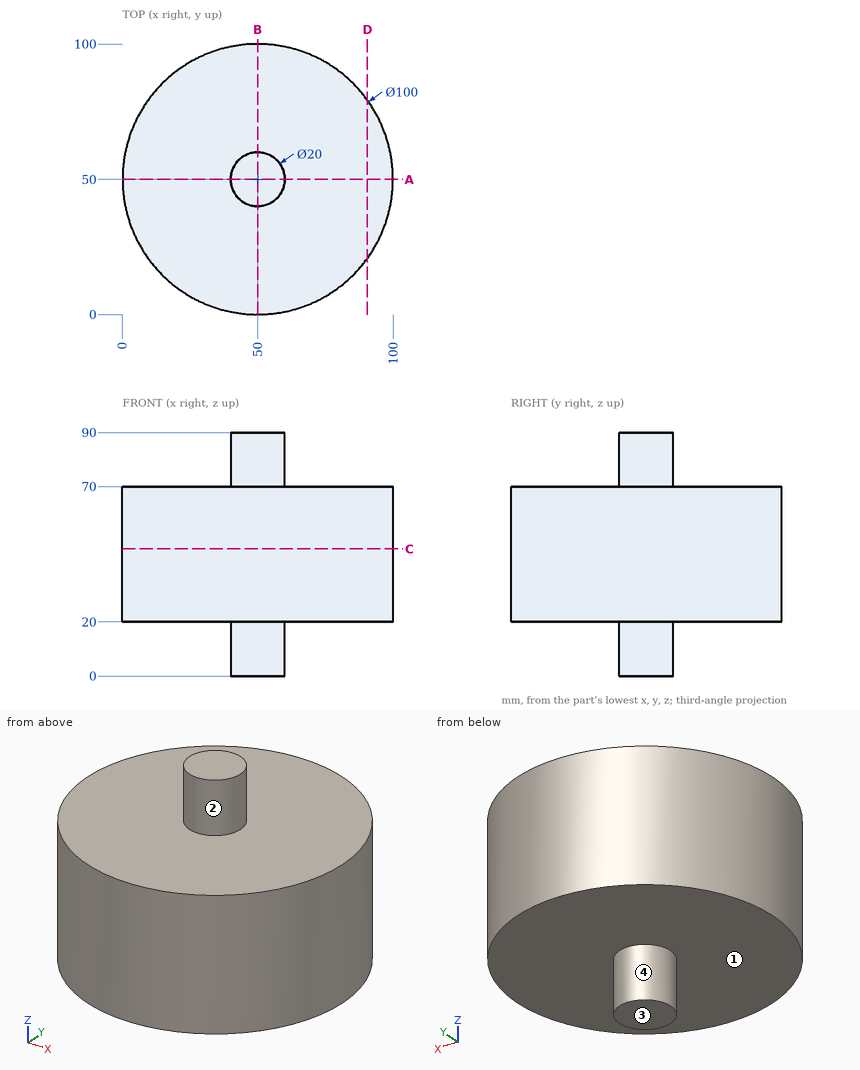
Verification items for this drawing (mm, ordinates from the low corner). A direction names the side the tool comes from. Give positions to 0.01 mm unless a question says otherwise; leave off trailing zeros. Loops run counter-clockwise (first coordinate to the right, second up) from the corner with the lowest first, then second, coordinate; pieces in that order, holes last. Notation, with made-up numbers: M 39.25,-37 L 48.25,-37 A12 ccw 48.25,-17 Z; hole C -19.75,39 d6. An arc over 180 degrees is marked long. Write item = value, one per line. Start each with the question number.
1. Draft check along X on the marked faces 1 and 2. Enter one of: +X half, -X half, draft (parallel to the pull), parting line (faces both ways), or undercut.
2. Section check C-C, the plane z = 47. Enter the section's corners in (x, y).
3. Tool access check on the marked faces 3 and 4. Record the directions out of +Z, -Z, +X, -X, +Y, -Y that give a thin tool (end or side, any length) a straight path to the whole face; none if there is none.
4. Section check D-D, the plane x = 90.5. Enter the section's corners in (y, z), plus the area to 3 significant figures.
5. Thickness scan on probe 1 along Z at (x, y) = (24, 12); probe 2 along Y at (x, z) = (23, 28.5); probe 3 along Y at (x, z) = (48, 51.5). Record the ranges inside material, lowest first.
6. Section check A-A, the plane y = 50. Enter the section's corners in (x, z).
7. Go/stop test with flat-tipped pins: P1, Ø4, axis at y = 65.5, z = 62, coming from the -X side; P2, Ø5, axis at x = 54, z = 65.5, coming from the +Y side; P3, Ø12, axis at x = 68, z = 18, coming from the -Y side. Record where each tip stops, or that it passes through.
Values follow:
q1.face_1 = draft
q1.face_2 = parting line
q2.outline = C 50,50 d100
q3.face_3 = -Z, +X, -X, +Y, -Y
q3.face_4 = -Z
q4.outline = M 20.68,20 L 79.32,20 L 79.32,70 L 20.68,70 Z
q4.area = 2,930 mm^2
q5.probe_1 = 20 to 70
q5.probe_2 = 7.92 to 92.08
q5.probe_3 = 0.04 to 99.96
q6.outline = M 0,20 L 40,20 L 40,0 L 60,0 L 60,20 L 100,20 L 100,70 L 60,70 L 60,90 L 40,90 L 40,70 L 0,70 Z
q7.P1 = 1.86
q7.P2 = 99.98
q7.P3 = 1.55
